Source: CAD feature listing. Evaluate the final solid. Frame: model axes, mm. Face numbers are marked on the shaded views. A direction names the side the tool comes from. Give positions to 0.01 mm unless a question says otherwise; leave off trailing zeros. Write each loop counter-clockwise with the first axis right and the second up, starting at its lowest first coordinate (ties: lowest second). Pieces come first, ordered by that corner, then holes. Notation, with made-up numbers: M 51.25,-24.5 L 84.25,-24.5 A36 cw 84.25,11.5 Z; hole C 8.5,-12 d6. An arc over 180 degrees is marked long. Return JSON: item names as keys, results as strings.
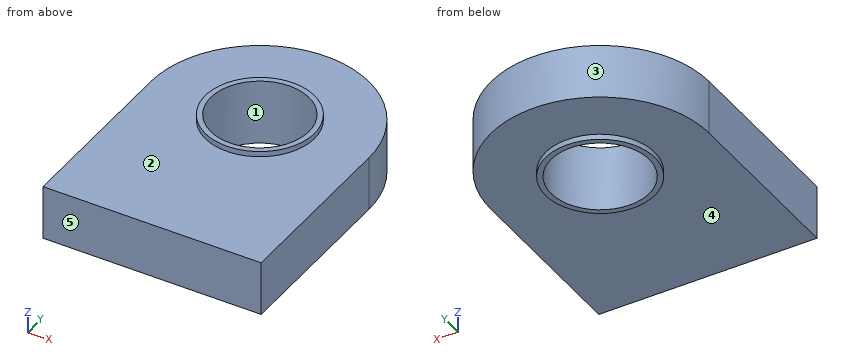
```python
from build123d import *

# Parameters (mm, degrees)
CROQUIS1_R                   = 4.5
SALIENTE_EXTRUIR1_DEPTH      = 5
SALIENTE_EXTRUIR3_DEPTH      = 3
SALIENTE_EXTRUIR3_DEPTH_BACK = 3
CROQUIS2_R                   = 5
CROQUIS2_R_2                 = 4.5


with BuildPart() as part:
    # Croquis1 → Saliente-Extruir1 (new body)
    with BuildSketch(Plane.XY):
        with BuildLine():
            Line((0, 0), (0, 16.5))
            ThreePointArc((0, 16.5), (10, 26.5), (20, 16.5))
            Line((20, 16.5), (20, 0))
            Line((20, 0), (0, 0))
        make_face()
        with Locations((10, 16.5)):
            Circle(CROQUIS1_R, mode=Mode.SUBTRACT)
    extrude(amount=SALIENTE_EXTRUIR1_DEPTH)

    # Croquis2 → Saliente-Extruir3 (add, two sides: drawn at the far end of the back side and taken through both)
    with BuildSketch(Plane.XY.offset(2.5).offset(-SALIENTE_EXTRUIR3_DEPTH_BACK)):
        with Locations((10, 16.5)):
            Circle(CROQUIS2_R)
        with Locations((10, 16.5)):
            Circle(CROQUIS2_R_2, mode=Mode.SUBTRACT)
    extrude(amount=SALIENTE_EXTRUIR3_DEPTH + SALIENTE_EXTRUIR3_DEPTH_BACK)


solid = part.part
```
1) Cut plane C-C, the plane x = 6.75. Return the cut outline in (y, z).
Numbers:
{"outline": "M 0,0 L 12.7,0 L 12.7,-0.5 L 13.39,-0.5 L 13.39,5.5 L 12.7,5.5 L 12.7,5 L 0,5 Z; M 19.61,-0.5 L 20.3,-0.5 L 20.3,0 L 25.96,0 L 25.96,5 L 20.3,5 L 20.3,5.5 L 19.61,5.5 Z"}
2) Contact query for a flat-ended pin moving along its axis: pin 1 Ø7 at (x, y) = (10, 16.5) entering from +Z. Output: stop coordinate, or through.
Numbers:
{"pin 1": "passes through"}
3) Line query: line 1 (Y direction, x = 10, z = 2.35); line 2 (Z direction, x = 9.75, y = 9); line 3 (X direction, y = 15.75, z = 4.3). Output: solid intervals per line, ascending. Write a range as [from, to].
Numbers:
{"line 1": "y = [0, 12], [21, 26.5]", "line 2": "z = [0, 5]", "line 3": "x = [0, 5.56], [14.44, 20]"}
4) Cut plane D-D, the plane y = 6.25. Return the cut outline in (x, z), then the cut area to 3 significant figures.
Numbers:
{"outline": "M 0,0 L 20,0 L 20,5 L 0,5 Z", "area": "100 mm²"}
5) Cut plane B-B, the plane z = 2.6. Return the cut outline in (x, y).
Numbers:
{"outline": "M 0,0 L 20,0 L 20,16.5 A10 ccw 0,16.5 Z; hole C 10,16.5 d9"}
6) Set-up query: the marked faces 4 and 5. Return all of +Z, -Z, +X, -X, +Y, -Y with unobstructed straight access to the full face (end or side cutting, diameter ignored); none if empty.
Numbers:
{"face 4": "-Z", "face 5": "+Z, -Z, +X, -X, -Y"}
7) Draft query along Y for the marked faces 1, 2 and 3. Return one class per face: released by +Y, released by -Y, zero draft, split by the parting line, or undercut.
Numbers:
{"face 1": "undercut", "face 2": "zero draft", "face 3": "released by +Y"}
8) Cut plane A-A, the plane x = 10. Return the cut outline in (y, z).
Numbers:
{"outline": "M 0,0 L 11.5,0 L 11.5,-0.5 L 12,-0.5 L 12,5.5 L 11.5,5.5 L 11.5,5 L 0,5 Z; M 21,-0.5 L 21.5,-0.5 L 21.5,0 L 26.5,0 L 26.5,5 L 21.5,5 L 21.5,5.5 L 21,5.5 Z"}
